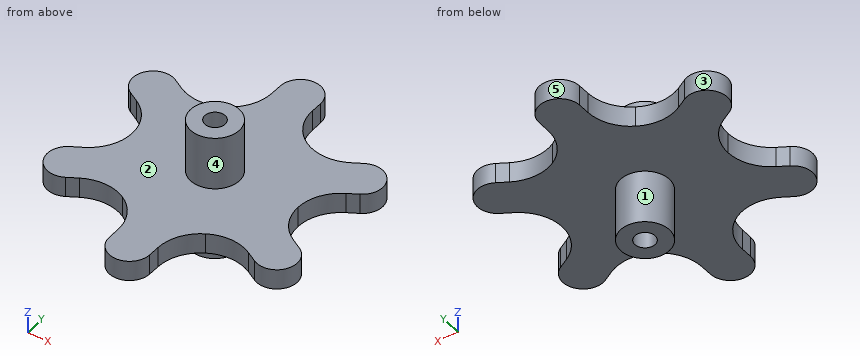
from build123d import *

# Parameters (mm, degrees)
F1_DEPTH = 1
F2_COUNT = 6
F3_R     = 2.4
F4_DEPTH = 6.25
F5_R     = 1
F6_DEPTH = 12.501


with BuildPart() as f1:
    # F0 (on Top) → F1 (new body, symmetric)
    with BuildSketch(Plane.XY):
        with BuildLine():
            Line((2, 10.8452994616), (2, 12))
            ThreePointArc((2, 12), (0, 14), (-2, 12))
            Line((-2, 12), (-2, 10.8452994616))
            ThreePointArc((-2, 10.8452994616), (-2.5709376404, 8.7145311798), (-4.1307682818, 7.1547005384))
            Line((-4.1307682818, 7.1547005384), (0, 0))
            Line((0, 0), (4.1307682818, 7.1547005384))
            ThreePointArc((4.1307682818, 7.1547005384), (2.5709376404, 8.7145311798), (2, 10.8452994616))
        make_face()
    extrude(amount=F1_DEPTH, both=True)

    # F2: F1 ×6 about axis
    f2_axis = Axis((0, 0, 0), (0, 0, -1))


with BuildPart() as f1_1:
    add(f1.part)
    for i in range(1, F2_COUNT):
        add(f1.part.rotate(f2_axis, i * 360 / F2_COUNT))

    # F3 (on Top) → F4 (join, symmetric)
    with BuildSketch(Plane.XY):
        Circle(F3_R)
    extrude(amount=F4_DEPTH, both=True)

    # F5 (on face) → F6 (cut, through all)
    with BuildSketch(Plane.XY.offset(6.25)):
        Circle(F5_R)
    extrude(amount=-F6_DEPTH, mode=Mode.SUBTRACT)


solid = f1_1.part
Geometry: final body of the model. Coordinates: model frame, mm. Face numbers are marked on the shaded views. A direction names the side the tool comes from. Give positions to 0.01 mm unless a question says otherwise; leave off trailing zeros. Write each loop counter-clockwise with the first axis right and the second up, starting at its lowest first coordinate (ties: lowest second). Pieces come first, ordered by that corner, then holes.
(1) Access query for the marked faces 4 and 5. Directions: +Z, -Z, +X, -X, +Y, -Y. A direction counts if a zero-diameter tool reaches every point of the face in a straight line with its end or side. Return the directions, or none.
(2) Ray query, line 1 (Y direction, x = 0, z = 2); line 2 (Z direction, x = 4.25, y = -3.5). Return the intervals inside material, ascending.
(3) Cut plane A-A, the plane x = 0. Return loops of the section in (y, z).
(4) Cut plane B-B, the plane z = -4. Return loops of the section in (x, y).
(5) Cut plane D-D, the plane y = 6. Return loops of the section in (x, z), then the cut area to 3 significant figures.
(6) First-contact query: P1, Ø12.5, axis at x = -6, y = -6.5, coming from the +Z side; P2, Ø1.3, axis at y = 11.5, z = 0, coming from the +X side; P3, Ø0.6, axis at y = -11.5, z = -0.5, coming from the -X side. Flat tips, straight axial feed; report the tip coordinate or a pass-through.
(7) Cut plane C-C, the plane x = -8.75. Return loops of the section in (y, z).
(8) Mould query, pull axis X, two halves, no side actions, for the marked faces 1, 2 and 3. Classes: released by +X, released by -X, zero draft, split by the parting line, or undercut.
Values follow:
1. face 4: +Z
1. face 5: +Z, -Z, +Y
2. line 1: y = -2.4 to -1, 1 to 2.4
2. line 2: z = -1 to 1
3. outline: (-14, -1) - (-2.4, -1) - (-2.4, -6.25) - (-1, -6.25) - (-1, 6.25) - (-2.4, 6.25) - (-2.4, 1) - (-14, 1) - close; (1, -6.25) - (2.4, -6.25) - (2.4, -1) - (14, -1) - (14, 1) - (2.4, 1) - (2.4, 6.25) - (1, 6.25) - close
4. outline: circle Ø4.8 at (0, 0); hole circle Ø2 at (0, 0)
5. outline: (-12.39, -1) - (12.39, -1) - (12.39, 1) - (-12.39, 1) - close
5. area: 49.6 mm2
6. P1: stops at z = 1
6. P2: stops at x = 2
6. P3: stops at x = -2
7. outline: (-7.36, -1) - (-1.98, -1) - (-1.98, 1) - (-7.36, 1) - close; (1.98, -1) - (7.36, -1) - (7.36, 1) - (1.98, 1) - close
8. face 1: split by the parting line
8. face 2: zero draft
8. face 3: undercut
